Design review of the part shown in the three views and the two pictorial views. Dimensions are in mm from the part's minimum x, y and z. A direction names the side the tool comes from. Round coordinates to 2 decimals unless told otherwise and drop trailing zeros. Order: outer loops, then holes, each group sorted by start corner. A loop starts at its lowest first (then second) coordinate and runs counter-clockwise, first axis right, second up.
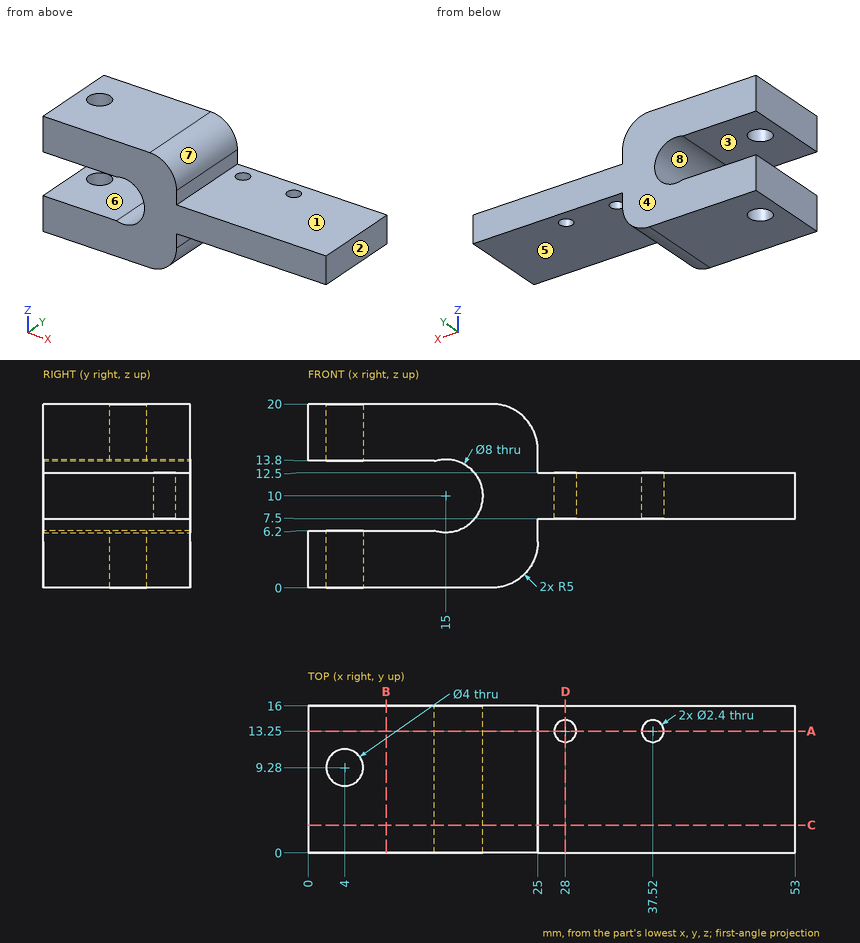
1) For the marked faces 1, 2, 3, 4 and 5, list the 3-axis set-ups (+Z, -Z, +X, -X, +Y, -Y) from which the entire face can be reached by the end or side of a thin tool; tool diameter is ignored.
Results:
face 1: +Z, +X, +Y, -Y
face 2: +Z, -Z, +X, +Y, -Y
face 3: -X, +Y, -Y
face 4: +Z, -Z, +X, -X, +Y
face 5: -Z, +X, +Y, -Y
2) To check wall thickness, follow line 1 along Z through (x, y) = (7, 15.75); line 2 along Y through (x, z) = (4, 4); line 3 along Y through (x, z) = (37.52, 9.55). State the ranges of each line that lie inside material, in increasing order.
Results:
line 1: z = 0 to 6.2, 13.8 to 20
line 2: y = 0 to 7.28, 11.28 to 16
line 3: y = 0 to 12.05, 14.45 to 16
3) Clearance check with flat-ended pins moving along their axes: P1, Ø1.3, axis at y = 11.5, z = 13.5, coming from the +X side; P2, Ø1.5, axis at x = 44, y = 9, coming from the -Z side; P3, Ø5, axis at x = 15, z = 10, coming from the +Y side; P4, Ø4, axis at x = 37.52, y = 13.25, coming from the +Z side. State where each tip first meets the part, or that it passes through.
Results:
P1: stops at x = 25
P2: stops at z = 7.5
P3: passes through
P4: stops at z = 12.5
4) Take a section at C-C on y = 3. Give the boundary of the cut face in (x, z).
Results:
outline: (0, 0) - (20, 0) arc R5 ccw to (25, 5) - (25, 7.5) - (53, 7.5) - (53, 12.5) - (25, 12.5) - (25, 15) arc R5 ccw to (20, 20) - (0, 20) - (0, 13.8) - (13.75, 13.8) arc R4 cw (long way) to (13.75, 6.2) - (0, 6.2) - close
5) Take a section at B-B on x = 8.5. Give the boundary of the cut face in (y, z), plus the area to 3 significant figures.
Results:
outline: (0, 0) - (16, 0) - (16, 6.2) - (0, 6.2) - close; (0, 13.8) - (16, 13.8) - (16, 20) - (0, 20) - close
area: 198 mm2
6) The part is to be moulded in two halves that separate along X. For the marked faces 6, 7 and 8, say which applies: released by +X, released by -X, zero draft, split by the parting line, or undercut.
Results:
face 6: zero draft
face 7: released by +X
face 8: undercut
7) Take a section at D-D on x = 28. Give the boundary of the cut face in (y, z), plus the area to 3 significant figures.
Results:
outline: (0, 7.5) - (12.05, 7.5) - (12.05, 12.5) - (0, 12.5) - close; (14.45, 7.5) - (16, 7.5) - (16, 12.5) - (14.45, 12.5) - close
area: 68.0 mm2
8) Take a section at A-A on y = 13.25. Give the boundary of the cut face in (x, z), plus the area to 3 significant figures.
Results:
outline: (0, 0) - (20, 0) arc R5 ccw to (25, 5) - (25, 7.5) - (26.8, 7.5) - (26.8, 12.5) - (25, 12.5) - (25, 15) arc R5 ccw to (20, 20) - (0, 20) - (0, 13.8) - (13.75, 13.8) arc R4 cw (long way) to (13.75, 6.2) - (0, 6.2) - close; (29.2, 7.5) - (36.32, 7.5) - (36.32, 12.5) - (29.2, 12.5) - close; (38.72, 7.5) - (53, 7.5) - (53, 12.5) - (38.72, 12.5) - close
area: 466 mm2
